Can you work these out from the model? Positions are in its coordinate system, mm. Face numbers are marked on the shaded views. A direction names the side the tool comes from. Give positions to 0.01 mm unless a question says otherwise; leave off trailing zeros. Write each loop counter-clockwise with the first axis right and the second up, starting at its lowest first coordinate (ties: lowest second). Pieces come first, ordered by that corner, then holes.
```python
from build123d import *

# Parameters (mm, degrees)
BOSS_EXTRUDE1_DEPTH = 631.317


with BuildPart() as part:
    # Sketch1 → Boss-Extrude1 (new body)
    with BuildSketch(Plane(origin=(0, 0, 0), x_dir=(1, 0, 0), z_dir=(0, 1, 0))):
        with BuildLine():
            Line((-38.1, -22.225), (-33.782, -22.225))
            Line((-33.782, -22.225), (-33.782, 13.589))
            ThreePointArc((-33.782, 13.589), (-32.517287081, 16.642287081), (-29.464, 17.907))
            Line((-29.464, 17.907), (29.464, 17.907))
            ThreePointArc((29.464, 17.907), (32.517287081, 16.642287081), (33.782, 13.589))
            Line((33.782, 13.589), (33.782, -22.225))
            Line((33.782, -22.225), (38.1, -22.225))
            Line((38.1, -22.225), (38.1, 17.907))
            ThreePointArc((38.1, 17.907), (36.835287081, 20.960287081), (33.782, 22.225))
            Line((33.782, 22.225), (-33.782, 22.225))
            ThreePointArc((-33.782, 22.225), (-36.835287081, 20.960287081), (-38.1, 17.907))
            Line((-38.1, 17.907), (-38.1, -22.225))
        make_face()
    extrude(amount=BOSS_EXTRUDE1_DEPTH)


solid = part.part
```
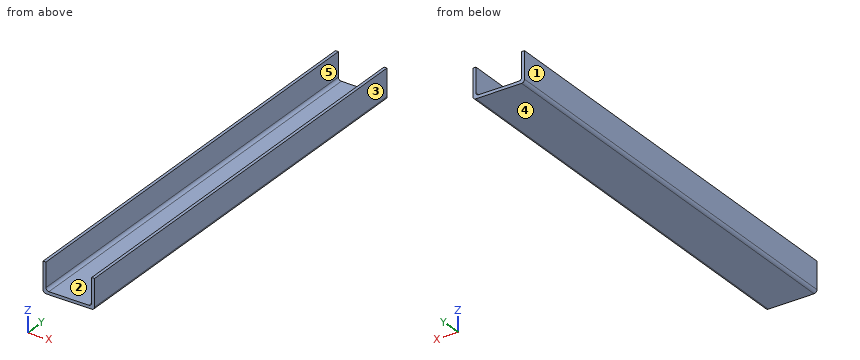
1) Suppose I cut it at B-B on y = 479.5. Write out the boundary of the cut face in (x, z) (3 decimals), plus the area to 3 significant figures.
Values follow:
outline: (-38.1, -17.907) arc R4.318 ccw to (-33.782, -22.225) - (33.782, -22.225) arc R4.318 ccw to (38.1, -17.907) - (38.1, 22.225) - (33.782, 22.225) - (33.782, -13.589) arc R4.318 cw to (29.464, -17.907) - (-29.464, -17.907) arc R4.318 cw to (-33.782, -13.589) - (-33.782, 22.225) - (-38.1, 22.225) - close
area: 676 mm2
2) If we mould it in two halves opening along X, with no side actions, what happens to the marked faces 1, 2 and 3? For each: +X half, -X half, draft (parallel to the pull), parting line (faces both ways), or undercut.
Values follow:
face 1: -X half
face 2: undercut
face 3: +X half
3) For pin 1 Ø10 at (x, z) = (24.5, -9) entering from -Y, with a flat end and sliding along its axis, tell me the tip position at first contact or that it passes through.
Values follow:
pin 1: passes through
4) Please list where these lines run through material, in increasing order: L1, parallel to X at y = 52, z = -9.5; L2, parallel to Z at x = 8, y = 154.5 (3 decimals); L3, parallel to X at y = 342, z = -17.
Values follow:
L1: x = -38.1 to -33.78, 33.78 to 38.1
L2: z = -22.225 to -17.907
L3: x = -38.1 to -32.11, 32.11 to 38.1
5) Suppose I cut it at C-C on x = 22.5. Write out the boundary of the cut face in (y, z) (3 decimals).
Values follow:
outline: (0, -22.225) - (631.317, -22.225) - (631.317, -17.907) - (0, -17.907) - close
6) For the marked faces 4 and 5, which set-ups out of +Z, -Z, +X, -X, +Y, -Y let a thin tool reach every point of the face, with its end or its side?
Values follow:
face 4: -Z, +X, -X, +Y, -Y
face 5: +Z, +Y, -Y
7) Suppose I cut it at A-A on z = 4.5. Write out the boundary of the cut face in (x, y).
Values follow:
outline: (-38.1, 0) - (-33.78, 0) - (-33.78, 631.32) - (-38.1, 631.32) - close; (33.78, 0) - (38.1, 0) - (38.1, 631.32) - (33.78, 631.32) - close
